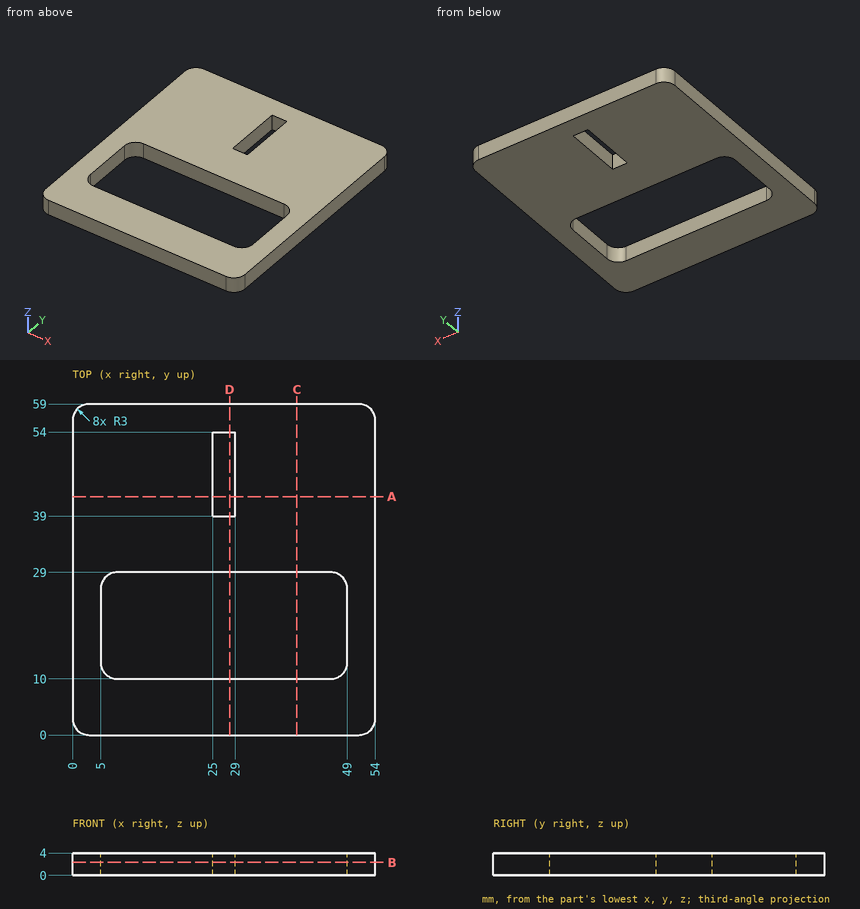
Check sheet for the drawn part. Datum: minimum x, y, z corner. Units: mm. Coordinates: 2 decimals unless noted, no trailing zeros. Order: outer loops, then holes, each group sorted by start corner. A loop starts at its lowest first (then second) coordinate and runs counter-clockwise, first axis right, second up. Notation, with made-up numbers: M 0,-25.75 L 52,-25.75 A28 cw 52,11.25 Z; hole C 17.25,51 d10. An arc over 180 degrees is marked long. One line per item, written item: value. Start each with the question number.
Item 1: Scan lines: probe 1 along Y at (x, z) = (27, 2.6); probe 2 along Y at (x, z) = (37, 1.65); probe 3 along X at (y, z) = (47, 2). Record each from-to range of solid material in increasing order.
Item 2: Sectioned sample at C-C (x = 40). Enter the section's corners in (y, z).
Item 3: Sectioned sample at A-A (y = 42.5). Enter the section's corners in (x, z), then the cut area to 3 significant figures.
Item 4: Sectioned sample at B-B (z = 2.35). Enter the section's corners in (x, y), then the cut area to 3 significant figures.
Item 5: Sectioned sample at D-D (x = 28). Enter the section's corners in (y, z), then the cut area to 3 significant figures.
Conclusion:
1. probe 1: y = 0 to 10, 29 to 39, 54 to 59
1. probe 2: y = 0 to 10, 29 to 59
1. probe 3: x = 0 to 25, 29 to 54
2. outline: M 0,0 L 10,0 L 10,4 L 0,4 Z; M 29,0 L 59,0 L 59,4 L 29,4 Z
3. outline: M 0,0 L 25,0 L 25,4 L 0,4 Z; M 29,0 L 54,0 L 54,4 L 29,4 Z
3. area: 200 mm^2
4. outline: M 0,3 A3 ccw 3,0 L 51,0 A3 ccw 54,3 L 54,56 A3 ccw 51,59 L 3,59 A3 ccw 0,56 Z; hole M 5,13 A3 ccw 8,10 L 46,10 A3 ccw 49,13 L 49,26 A3 ccw 46,29 L 8,29 A3 ccw 5,26 Z; hole M 25,39 L 29,39 L 29,54 L 25,54 Z
4. area: 2,290 mm^2
5. outline: M 0,0 L 10,0 L 10,4 L 0,4 Z; M 29,0 L 39,0 L 39,4 L 29,4 Z; M 54,0 L 59,0 L 59,4 L 54,4 Z
5. area: 100 mm^2
